from build123d import *

# Parameters (mm, degrees)
F0_R     = 11.2
F1_DEPTH = 7
F3_DEPTH = 7


with BuildPart() as f1:
    # F0 (on Top) → F1 (new body)
    with BuildSketch(Plane.XY):
        with BuildLine():
            ThreePointArc((10.1597440205, 17.8761330961), (12.4166948314, 21.8239716806), (13.2, 26.3034459203))
            ThreePointArc((13.2, 26.3034459203), (-5.5373555744, 38.2858368855), (-8.5541959459, 16.2503005558))
            ThreePointArc((-8.5541959459, 16.2503005558), (-5.0829218379, 14.1213317529), (-1.12791098, 13.1517229602))
            ThreePointArc((-1.12791098, 13.1517229602), (0, 13.2), (1.12791098, 13.1517229602))
            ThreePointArc((1.12791098, 13.1517229602), (6.1182351733, 14.606984987), (10.1597440205, 17.8761330961))
        make_face()
        with Locations((0, 26.3034459203)):
            Circle(F0_R, mode=Mode.SUBTRACT)
        with BuildLine():
            ThreePointArc((-1.12791098, 13.1517229602), (-5.0829218379, 14.1213317529), (-8.5541959459, 16.2503005558))
            ThreePointArc((-8.5541959459, 16.2503005558), (-9.0756063849, 11.8077563343), (-10.7501080818, 7.6599723387))
            ThreePointArc((-10.7501080818, 7.6599723387), (-6.5430623893, 11.4642197541), (-1.12791098, 13.1517229602))
        make_face()
        with BuildLine():
            ThreePointArc((11.3058248826, 6.8130994213), (9.7913703879, 12.2470899677), (10.1597440205, 17.8761330961))
            ThreePointArc((10.1597440205, 17.8761330961), (6.1182351733, 14.606984987), (1.12791098, 13.1517229602))
            ThreePointArc((1.12791098, 13.1517229602), (6.9781074775, 11.204731859), (11.3058248826, 6.8130994213))
        make_face()
        with BuildLine():
            ThreePointArc((1.12791098, 13.1517229602), (0, 13.2), (-1.12791098, 13.1517229602))
            ThreePointArc((-1.12791098, 13.1517229602), (0, 13.1034459203), (1.12791098, 13.1517229602))
        make_face()
        with BuildLine():
            ThreePointArc((1.12791098, 13.1517229602), (0, 13.1034459203), (-1.12791098, 13.1517229602))
            ThreePointArc((-1.12791098, 13.1517229602), (-6.5430623893, 11.4642197541), (-10.7501080818, 7.6599723387))
            ThreePointArc((-10.7501080818, 7.6599723387), (-11.1373686058, 7.0132721384), (-11.5532296186, 6.3845818484))
            ThreePointArc((-11.5532296186, 6.3845818484), (-13.1926361713, 0.4408524163), (-11.9536816771, -5.5990619182))
            ThreePointArc((-11.9536816771, -5.5990619182), (-11.3479170441, -6.5517229602), (-10.825770697, -7.552661042))
            ThreePointArc((-10.825770697, -7.552661042), (-6.6567743469, -11.3985681247), (-1.2586765967, -13.1398528616))
            ThreePointArc((-1.2586765967, -13.1398528616), (-0.5049875326, -13.1518802131), (0.247404736, -13.1976812697))
            ThreePointArc((0.247404736, -13.1976812697), (6.2145286938, -11.6455842754), (10.825770697, -7.552661042))
            ThreePointArc((10.825770697, -7.552661042), (11.3479170441, -6.5517229602), (11.9536816771, -5.5990619182))
            ThreePointArc((11.9536816771, -5.5990619182), (12.8846536263, -2.8680482791), (13.2, 0))
            ThreePointArc((13.2, 0), (12.8987588115, 2.8039295858), (12.0087846785, 5.4798805229))
            ThreePointArc((12.0087846785, 5.4798805229), (11.6423561384, 6.1386080748), (11.3058248826, 6.8130994213))
            ThreePointArc((11.3058248826, 6.8130994213), (6.9781074775, 11.204731859), (1.12791098, 13.1517229602))
        make_face()
        Circle(F0_R, mode=Mode.SUBTRACT)
        with BuildLine():
            ThreePointArc((12.0087846785, 5.4798805229), (11.6763488687, 6.1565312552), (11.3058248826, 6.8130994213))
            ThreePointArc((11.3058248826, 6.8130994213), (11.6423561384, 6.1386080748), (12.0087846785, 5.4798805229))
        make_face()
        with BuildLine():
            ThreePointArc((-11.9536816771, -5.5990619182), (-13.1926361713, 0.4408524163), (-11.5532296186, 6.3845818484))
            ThreePointArc((-11.5532296186, 6.3845818484), (-15.5019762284, 2.35603051), (-20.5610573929, -0.1394701303))
            ThreePointArc((-20.5610573929, -0.1394701303), (-15.7091376581, -2.0049454071), (-11.9536816771, -5.5990619182))
        make_face()
        with BuildLine():
            ThreePointArc((18.3502710734, -0.7169992799), (14.7636201396, 1.955827517), (12.0087846785, 5.4798805229))
            ThreePointArc((12.0087846785, 5.4798805229), (12.8987588115, 2.8039295858), (13.2, 0))
            ThreePointArc((13.2, 0), (12.8846536263, -2.8680482791), (11.9536816771, -5.5990619182))
            ThreePointArc((11.9536816771, -5.5990619182), (14.7708929522, -2.6587264394), (18.3502710734, -0.7169992799))
        make_face()
        with BuildLine():
            ThreePointArc((-10.825770697, -7.552661042), (-11.3479170441, -6.5517229602), (-11.9536816771, -5.5990619182))
            ThreePointArc((-11.9536816771, -5.5990619182), (-11.43153533, -6.6), (-10.825770697, -7.552661042))
        make_face()
        with BuildLine():
            ThreePointArc((-10.825770697, -7.552661042), (-11.43153533, -6.6), (-11.9536816771, -5.5990619182))
            ThreePointArc((-11.9536816771, -5.5990619182), (-15.7091376581, -2.0049454071), (-20.5610573929, -0.1394701303))
            ThreePointArc((-20.5610573929, -0.1394701303), (-33.5968448072, -20.7163789966), (-9.7960751276, -15.533301276))
            ThreePointArc((-9.7960751276, -15.533301276), (-9.633719613, -14.3474278455), (-9.5794523741, -13.1517229602))
            ThreePointArc((-9.5794523741, -13.1517229602), (-9.8947987478, -10.283674681), (-10.825770697, -7.552661042))
        make_face()
        with Locations((-22.7794523741, -13.1517229602)):
            Circle(F0_R, mode=Mode.SUBTRACT)
        with BuildLine():
            ThreePointArc((35.9794523741, -13.1517229602), (30.3878295608, -2.3650368804), (18.3502710734, -0.7169992799))
            ThreePointArc((18.3502710734, -0.7169992799), (14.7708929522, -2.6587264394), (11.9536816771, -5.5990619182))
            ThreePointArc((11.9536816771, -5.5990619182), (11.43153533, -6.6), (10.825770697, -7.552661042))
            ThreePointArc((10.825770697, -7.552661042), (9.5909024848, -12.6020395799), (10.4013133724, -17.7366629658))
            ThreePointArc((10.4013133724, -17.7366629658), (25.1084613025, -26.1446332351), (35.9794523741, -13.1517229602))
        make_face()
        with Locations((22.7794523741, -13.1517229602)):
            Circle(F0_R, mode=Mode.SUBTRACT)
        with BuildLine():
            ThreePointArc((-1.2586765967, -13.1398528616), (-6.6567743469, -11.3985681247), (-10.825770697, -7.552661042))
            ThreePointArc((-10.825770697, -7.552661042), (-9.8947987478, -10.283674681), (-9.5794523741, -13.1517229602))
            ThreePointArc((-9.5794523741, -13.1517229602), (-9.633719613, -14.3474278455), (-9.7960751276, -15.533301276))
            ThreePointArc((-9.7960751276, -15.533301276), (-5.6880137547, -13.7635838512), (-1.2586765967, -13.1398528616))
        make_face()
        with BuildLine():
            ThreePointArc((10.825770697, -7.552661042), (11.43153533, -6.6), (11.9536816771, -5.5990619182))
            ThreePointArc((11.9536816771, -5.5990619182), (11.3479170441, -6.5517229602), (10.825770697, -7.552661042))
        make_face()
        with BuildLine():
            ThreePointArc((10.4013133724, -17.7366629658), (9.5909024848, -12.6020395799), (10.825770697, -7.552661042))
            ThreePointArc((10.825770697, -7.552661042), (6.2145286938, -11.6455842754), (0.247404736, -13.1976812697))
            ThreePointArc((0.247404736, -13.1976812697), (5.7106058405, -14.6031204777), (10.4013133724, -17.7366629658))
        make_face()
    extrude(amount=F1_DEPTH)

    # F2 (on Top) → F3 (join)
    with BuildSketch(Plane.XY):
        with BuildLine():
            ThreePointArc((12.2943036258, 4.9750674516), (15.5675466721, 11.6262977505), (20.9984593093, 6.580688525))
            ThreePointArc((20.9984593093, 6.580688525), (18.2353036168, 14.8413488661), (10.0971376523, 17.9467946291))
            ThreePointArc((10.0971376523, 17.9467946291), (9.9225536839, 11.2452805665), (12.2943036258, 4.9750674516))
        make_face()
        with BuildLine():
            ThreePointArc((-1.8386170143, -13.1347129876), (2.2848958678, -19.2950397679), (-4.8001862176, -21.4755434647))
            ThreePointArc((-4.8001862176, -21.4755434647), (3.735333336, -23.2129106109), (10.4938112391, -17.717775027))
            ThreePointArc((10.4938112391, -17.717775027), (4.7859075855, -14.1929896942), (-1.8386170143, -13.1347129876))
        make_face()
        with BuildLine():
            ThreePointArc((-10.4556866115, 8.159645536), (-17.85244254, 7.6687420174), (-16.1982730917, 14.8948549397))
            ThreePointArc((-16.1982730917, 14.8948549397), (-21.9706369528, 8.3715617448), (-20.5909488915, -0.2290196021))
            ThreePointArc((-20.5909488915, -0.2290196021), (-14.6756844073, 2.9411945739), (-10.4556866115, 8.159645536))
        make_face()
    extrude(amount=F3_DEPTH)


solid = f1.part
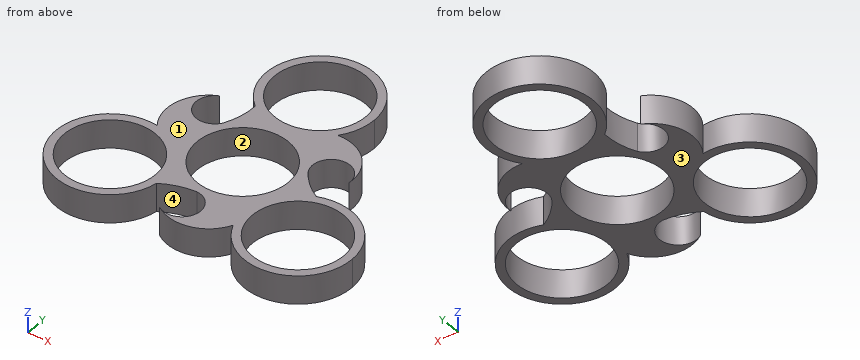
Verification items for the finished model (mm, model axes). Face numbers are marked on the shaded views. A direction names the side the tool comes from. Coordinates: 2 decimals unless noted, no trailing zeros. Write each loop counter-clockwise with the first axis right and the second up, starting at its lowest first coordinate (ties: lowest second). Pieces come first, ordered by that corner, then holes. Notation, with made-up numbers: (21.25, 50.25) - (27.25, 50.25) arc R22 cw to (27.25, 57.25) - close; hole circle Ø10 at (21, 78). An arc over 180 degrees is marked (long way). Answer as a JSON object with one key per item and string values.
(1) Cross-section at A-A on z = 1. Record the cut outline in (x, y), plus the area to 3 significant figures.
Report:
{"outline": "(-20.66, -0.12) arc R13.2 ccw (long way) to (-9.8, -15.53) arc R16.81 cw to (-1.66, -13.15) arc R4.62 cw (long way) to (-4.8, -21.48) arc R10.19 ccw to (10.44, -17.83) arc R13.2 ccw (long way) to (18.35, -0.72) arc R16.81 cw to (12.22, 5.14) arc R4.62 cw (long way) to (21, 6.58) arc R10.19 ccw to (10.23, 17.96) arc R13.2 ccw (long way) to (-8.55, 16.25) arc R16.81 cw to (-10.56, 8.01) arc R4.62 cw (long way) to (-16.2, 14.89) arc R10.19 ccw to start; hole circle Ø22.4 at (-22.78, -13.15); hole circle Ø22.4 at (0, 0); hole circle Ø22.4 at (0, 26.3); hole (10.09, 10.4) arc R16.81 ccw to (10.87, 7.83) arc R17.4 cw to start; hole circle Ø22.4 at (22.78, -13.15)", "area": "945 mm^2"}
(2) Tool access check on the marked faces 3 and 4. Record the directions out of +Z, -Z, +X, -X, +Y, -Y that give a thin tool (end or side, any length) a straight path to the whole face; none if there is none.
Report:
{"face 3": "-Z, +X, -X, +Y, -Y", "face 4": "+Z, -Z"}
(3) Thickness scan on line 1 along X through (y, z) = (26.5, 5); line 2 along Y through (x, z) = (18, 0.75); line 3 along Y through (x, z) = (6.5, 1.5). Record the ranges inside material, lowest first.
Report:
{"line 1": "-13.2 to -11.2, 11.2 to 13.2", "line 2": "-25.46 to -23.28, -3.02 to -0.52, 11.42 to 15.08", "line 3": "-22.08 to -9.12, 9.12 to 17.18, 35.42 to 37.79"}
(4) Mould release check, pull along Y, two halves, no side actions. Record for the marked faces 1 and 2: pulls with the +Y half, pulls with the -Y half, needs draft (parallel to the pull), parting line crosses it, or undercut.
Report:
{"face 1": "needs draft", "face 2": "undercut"}
(5) Gauge pin test, flat ends, axial feed: pin 1 Ø7.5 at (x, y) = (16.41, 7.08) entering from -Z; pin 2 Ø4 at (x, z) = (16.5, 1.5) entering from +Y; pin 3 Ø2 at (y, z) = (-0.5, 1) entering from +X. Record the tip position at first contact, or that the pin passes through.
Report:
{"pin 1": "through", "pin 2": "y = 17.31", "pin 3": "x = 28.98"}
(6) Cross-section at B-B on y = 25.5. Record the cut outline in (x, z).
Report:
{"outline": "(-13.18, 0) - (-11.17, 0) - (-11.17, 7) - (-13.18, 7) - close; (11.17, 0) - (13.18, 0) - (13.18, 7) - (11.17, 7) - close"}
(7) Cross-section at C-C on x = 0. Record the cut outline in (y, z).
Report:
{"outline": "(-23.42, 0) - (-21.88, 0) - (-21.88, 7) - (-23.42, 7) - close; (-13.62, 0) - (-11.2, 0) - (-11.2, 7) - (-13.62, 7) - close; (11.2, 0) - (15.1, 0) - (15.1, 7) - (11.2, 7) - close; (37.5, 0) - (39.5, 0) - (39.5, 7) - (37.5, 7) - close"}
